```python
from build123d import *

# Parameters (mm, degrees)
F0_W     = 120
F0_H     = 90
F1_DEPTH = 80
F2_R     = 5
F3_T     = -3
F5_DEPTH = 1


with BuildPart() as f1:
    # F0 (on Top) → F1 (new body)
    with BuildSketch(Plane.XY):
        Rectangle(F0_W, F0_H)
    extrude(amount=F1_DEPTH)

    # F2
    f2_edges = [f1.edges().sort_by_distance(p)[0] for p in [
        (60, -45, 40),
        (-60, -45, 40),
        (0, -45, 80),
        (60, 0, 80),
        (60, 45, 40),
        (0, 45, 80),
        (-60, 0, 80),
        (-60, 45, 40),
    ]]
    fillet(f2_edges, radius=F2_R)

    # F3
    f3_openings = [f1.faces().sort_by_distance(p)[0] for p in [
        (0, 0, 0),
    ]]
    offset(amount=F3_T, openings=f3_openings)

    # F4 (on face) → F5 (cut)
    with BuildSketch(Plane(origin=(0, 0, 0), x_dir=(1, 0, 0), z_dir=(0, 0, -1))):
        with BuildLine():
            ThreePointArc((58, 40), (57.12132, 42.12132), (55, 43))
            Line((55, 43), (-55, 43))
            ThreePointArc((-55, 43), (-57.12132, 42.12132), (-58, 40))
            Line((-58, 40), (-58, -40))
            ThreePointArc((-58, -40), (-57.12132, -42.12132), (-55, -43))
            Line((-55, -43), (55, -43))
            ThreePointArc((55, -43), (57.12132, -42.12132), (58, -40))
            Line((58, -40), (58, 40))
        make_face()
    extrude(amount=-F5_DEPTH, mode=Mode.SUBTRACT)


solid = f1.part
```
Verification items for the finished model (mm, model axes). A direction names the side the tool comes from. Coordinates: 2 decimals unless noted, no trailing zeros. Loops run counter-clockwise (first coordinate to the right, second up) from the corner with the lowest first, then second, coordinate; pieces in that order, holes last. Notation, with made-up numbers: (-35.5, -7.75) -> (2.5, -7.75) arc R24 ccw to (2.5, 5.25) -> close; hole circle Ø6 at (55.5, 49). An arc over 180 degrees is marked (long way). Put each result on its own line as item: value.
1. Gauge pin test, flat ends, axial feed: P1, Ø12, axis at x = -19.5, y = 35, coming from the -Z side; P2, Ø2, axis at x = -21, y = -9.5, coming from the -Z side. Record the tip position at first contact, or that the pin passes through.
Result set:
P1: stops at z = 76.73
P2: stops at z = 77
2. Thickness scan on line 1 (Y direction, x = -36.5, z = 12); line 2 (X direction, y = 10, z = 74); line 3 (Z direction, x = -44, y = -2). Record the ranges inside material, lowest first.
Result set:
line 1: y = -45 to -42, 42 to 45
line 2: x = -60 to -57, 57 to 60
line 3: z = 77 to 80
3. Tool access check on faces 1 (the face through (57.1, 42.14, 0.49)), 2 (the face through (59, 1, 78)). Record the directions out of +Z, -Z, +X, -X, +Y, -Y that give a thin tool (end or side, any length) a straight path to the whole face; none if there is none.
Result set:
face 1: -Z
face 2: +Z, +X, +Y, -Y
4. Mould release check, pull along Y, two halves, no side actions. Record for faces 3 (the face through (-57, -1, 37)), 4 (the face through (1, -44, 78)), 5 (the face through (-1, 1, 80)): pulls with the +Y half, pulls with the -Y half, needs draft (parallel to the pull), parting line crosses it, or undercut.
Result set:
face 3: undercut
face 4: pulls with the -Y half
face 5: needs draft
5. Section check A-A, the plane z = 21.5. Record the boundary of the cut face in (x, y).
Result set:
outline: (-60, -40) arc R5 ccw to (-55, -45) -> (55, -45) arc R5 ccw to (60, -40) -> (60, 40) arc R5 ccw to (55, 45) -> (-55, 45) arc R5 ccw to (-60, 40) -> close; hole (-57, -40) arc R2 ccw to (-55, -42) -> (55, -42) arc R2 ccw to (57, -40) -> (57, 40) arc R2 ccw to (55, 42) -> (-55, 42) arc R2 ccw to (-57, 40) -> close
6. Section check B-B, the plane y = 25. Record the boundary of the cut face in (x, z).
Result set:
outline: (-60, 0) -> (-58, 0) -> (-58, 1) -> (-57, 1) -> (-57, 75) arc R2 cw to (-55, 77) -> (55, 77) arc R2 cw to (57, 75) -> (57, 1) -> (58, 1) -> (58, 0) -> (60, 0) -> (60, 75) arc R5 ccw to (55, 80) -> (-55, 80) arc R5 ccw to (-60, 75) -> close
7. Section check C-C, the plane x = -41.5. Record the boundary of the cut face in (y, z), then the cut area to 3 significant figures.
Result set:
outline: (-45, 0) -> (-43, 0) -> (-43, 1) -> (-42, 1) -> (-42, 75) arc R2 cw to (-40, 77) -> (40, 77) arc R2 cw to (42, 75) -> (42, 1) -> (43, 1) -> (43, 0) -> (45, 0) -> (45, 75) arc R5 ccw to (40, 80) -> (-40, 80) arc R5 ccw to (-45, 75) -> close
area: 721 mm^2
